```python
from build123d import *

# Parameters (mm, degrees)
CYLINDER_R     = 12.5
CYLINDER_DEPTH = 8.068975


with BuildPart() as sphere001:
    # Sphere001 → Sphere001 (revolve)
    with BuildSketch(Plane(origin=(0, 0, -47.645512), x_dir=(1, 0, 0), z_dir=(0, -1, 0))):
        with BuildLine():
            ThreePointArc((0, -51.68), (51.68, 0), (0, 51.68))
            Line((0, 51.68), (0, -51.68))
        make_face()
    revolve(axis=Axis((0, 0, -47.645512), (0, 0, 1)))


with BuildPart() as common:
    # Sphere → Sphere (revolve)
    with BuildSketch(Plane(origin=(0, 0, 47.645512), x_dir=(1, 0, 0), z_dir=(0, -1, 0))):
        with BuildLine():
            ThreePointArc((0, -51.68), (51.68, 0), (0, 51.68))
            Line((0, 51.68), (0, -51.68))
        make_face()
    revolve(axis=Axis((0, 0, 47.645512), (0, 0, 1)))

    # Common: intersect Sphere001
    add(sphere001.part, mode=Mode.INTERSECT)


with BuildPart() as lens:
    # Cylinder → Cylinder (new body)
    with BuildSketch(Plane.XY.offset(-4.034488)):
        Circle(CYLINDER_R)
    extrude(amount=CYLINDER_DEPTH)

    # Common001: intersect Common
    add(common.part, mode=Mode.INTERSECT)


solid = lens.part
```
The model under review builds one solid part; all positions refer to its coordinate system, in mm. Round coordinates to 2 decimals unless told otherwise and drop trailing zeros. Loops run counter-clockwise (first coordinate to the right, second up) from the corner with the lowest first, then second, coordinate; pieces in that order, holes last.
Item 1: Take a section at A-A (z = 0). Write out the cut boundary in (x, y), then the cut area to 3 significant figures.
Determined:
outline: circle Ø25 at (0, 0)
area: 491 mm2
Item 2: Take a section at B-B (y = 10.75). Write out the cut boundary in (x, z), then the cut area to 3 significant figures.
Determined:
outline: (-6.38, -2.5) arc R50.55 ccw to (6.38, -2.5) - (6.38, 2.5) arc R50.55 ccw to (-6.38, 2.5) - close
area: 70.7 mm2
Item 3: For line 1 (X direction, y = -10.5, z = -2); line 2 (Z direction, x = 0, y = -7.5); line 3 (Y direction, x = -8, z = -2.25), list the stretches that pass through material, from the lowest coordinate up.
Determined:
line 1: x = -6.78 to 6.78
line 2: z = -3.49 to 3.49
line 3: y = -9.6 to 9.6
Item 4: Clearance check with flat-ended pins moving along their axes: pin 1 Ø8 at (x, y) = (-2, 9.5) entering from -Z; pin 2 Ø4 at (x, z) = (-7, 1.5) entering from +Y; pin 3 Ø8 at (x, y) = (-4.5, 7) entering from +Z. State where each tip first meets the part, or that it passes through.
Determined:
pin 1: stops at z = -3.72
pin 2: stops at y = 11.46
pin 3: stops at z = 3.85
